Job drawing, mm, ordinate dimensions from the low corner. One solid piece. Give positions to 0.01 mm unless a question says otherwise; leave off trailing zeros. Loops run counter-clockwise (first coordinate to the right, second up) from the corner with the lowest first, then second, coordinate; pieces in that order, holes last. Notation, with made-up numbers: (69.5, 69.5) - (126.5, 69.5) arc R16 cw to (126.5, 95.5) - close; hole circle Ø10 at (74, 81.25). An arc over 180 degrees is marked (long way). Answer as CSV lines item,"result". Start each with the question number.
Item 1: Saw through at A-A on y = 27.25. Give the cut face in (x, z).
Item 2: Drill centre lines: L1, parallel to X at y = 4.75, z = 4.55 (1 decimal); L2, parallel to X at y = 23.5, z = 2.7 (1 decimal); L3, parallel to Y at x = 59, z = 1.25 (1 decimal). Where is each one in solid material? Low to high. Write a range as from..to.
Item 3: Pin check, flat tip, straight feed: pin 1 (4.5 mm diameter, centred on x = 59.87, y = 4.04, fed in from +Z). Stop position of the tip, or through.
Item 4: Saw through at B-B on z = 4. Give the cut face in (x, y), plus the area to 3 significant figures.
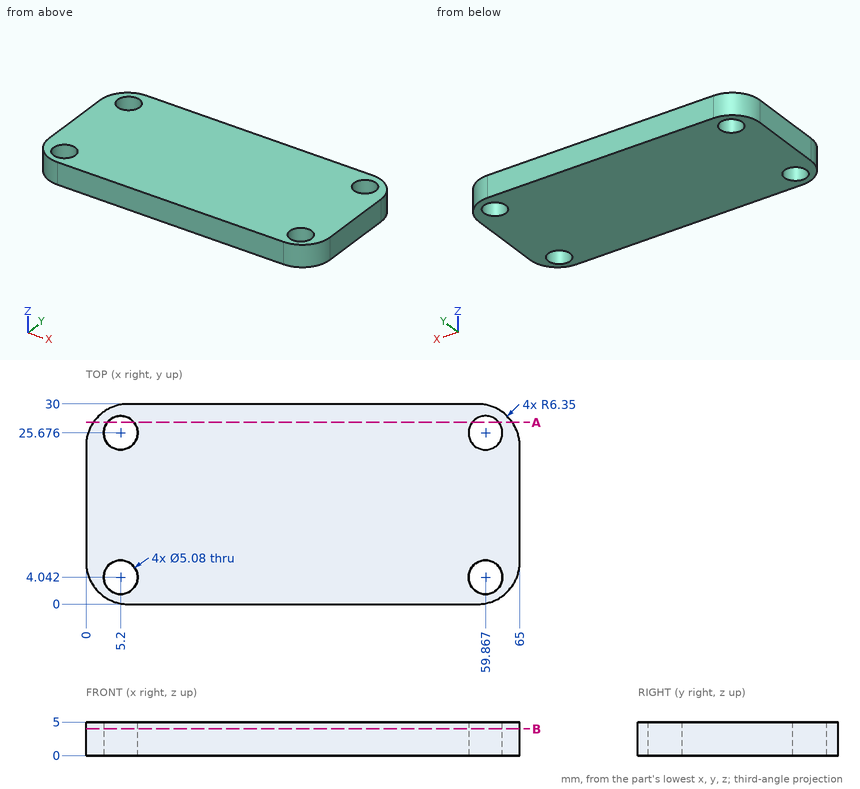
Responses:
1,outline,"(1.12, 0) - (3.21, 0) - (3.21, 5) - (1.12, 5) - close; (7.19, 0) - (57.87, 0) - (57.87, 5) - (7.19, 5) - close; (61.86, 0) - (63.88, 0) - (63.88, 5) - (61.86, 5) - close"
2,L1,"0.2..2.8, 7.6..57.4, 62.3..64.8"
2,L2,"0..3.9, 6.5..58.6, 61.2..65"
2,L3,"0..1.7, 6.4..23.3, 28.1..30"
3,pin 1,"through"
4,outline,"(0, 6.35) arc R6.35 ccw to (6.35, 0) - (58.65, 0) arc R6.35 ccw to (65, 6.35) - (65, 23.65) arc R6.35 ccw to (58.65, 30) - (6.35, 30) arc R6.35 ccw to (0, 23.65) - close; hole circle Ø5.08 at (5.2, 4.04); hole circle Ø5.08 at (5.2, 25.68); hole circle Ø5.08 at (59.87, 4.04); hole circle Ø5.08 at (59.87, 25.68)"
4,area,"1,830 mm2"
